Autodesk Inventor part; units mm, degrees
ref_plane "YZ Plane" through (0, 0, 0) normal (1, 0, 0) x (0, 1, 0)
ref_plane "XZ Plane" through (0, 0, 0) normal (0, 1, 0) x (-1, 0, 0)
ref_plane "XY Plane" through (0, 0, 0) normal (0, 0, 1) x (1, 0, 0)
sketch "スケッチ1" plane through (0, 0, 0) normal (0, 1, 0) x (-1, 0, 0)
  line L0 (7.5, -7.5) -> (-7.5, -7.5)
  line L1 (-7.5, -7.5) -> (-7.5, 7.5)
  line L2 (-7.5, 7.5) -> (7.5, 7.5)
  line L3 (7.5, 7.5) -> (7.5, -7.5)
  line L4 (7.5, -7.5) -> (-7.5, 7.5) construction
  line L5 (-7.5, -7.5) -> (7.5, 7.5) construction
  point P0 (0, 0)
  dimension "d0" = 15
  dimension "d1" = 15
extrude "押し出し1" add sketch "スケッチ1" along normal blind 140
shell "シェル1" thickness 1 removed faces 2 at (-2.5, 0, -2.5) at (-2.5, 140, -2.5)
sketch "スケッチ2" plane through (-7.5, 0, 7.5) normal (0, 0, 1) x (1, 0, 0)
  line L0 (15, 0) -> (0, 0)
  line L1 (0, 140) -> (15, 140)
  point P0 (7.5, 0)
  point P1 (7.5, 8)
  point P2 (7.5, 23)
  point P3 (7.5, 0)
  point P4 (7.5, 132)
  point P5 (7.5, 112)
  point P6 (7.5, 140)
  dimension "d5" = 8
  dimension "d6" = 15
  dimension "d14" = 8
  dimension "d15" = 20
hole "穴1" at (0, 8, 7.5) at (0, 23, 7.5) at (0, 132, 7.5) at (0, 112, 7.5) direction (0, 0, -1) diameter 3.2 end through all
sketch "スケッチ3" plane through (-7.5, 0, -7.5) normal (-1, 0, 0) x (0, 0, 1)
  line L0 (15, 0) -> (0, 0)
  point P0 (7.5, 0)
  point P1 (7.5, 37.5)
  point P2 (7.5, 102.5)
  point P3 (7.5, 0)
  point P4 (7.5, 0)
  dimension "d16" = 37.5
  dimension "d17" = 65
hole "穴2" at (-7.5, 37.5, 0) at (-7.5, 102.5, 0) direction (1, 0, 0) diameter 3.2 end through all
sketch "スケッチ4" plane through (-7.5, 0, 7.5) normal (0, 0, 1) x (1, 0, 0)
  circle A0 centre (94.8138, 137.4022) radius 1.6
  circle A1 centre (-2.6682, 183.8917) radius 1.6
  circle A2 centre (99.3065, 100.3608) radius 1.6
  circle A3 centre (1.8246, 146.8503) radius 1.6
  circle A4 centre (7.5, 112) radius 1.2295
  circle A5 centre (7.5, 132) radius 1.2295
  line L0 (112.2687, 136.8332) -> (109.5609, 138.1246)
  arc A6 (110.4218, 139.9298) -> (109.5609, 138.1246) centre (109.9914, 139.0272) ccw
  line L1 (110.4218, 139.9298) -> (112.1436, 143.5402)
  arc A7 (113.8704, 143.6762) -> (112.1436, 143.5402) centre (113.0463, 143.1098) ccw
  arc A8 (114.8515, 142.2489) -> (113.8704, 143.6762) centre (113.9489, 142.6793) ccw
  line L2 (114.8515, 142.2489) -> (113.1296, 138.6384)
  arc A9 (112.2687, 136.8332) -> (113.1296, 138.6384) centre (112.6992, 137.7358) ccw
  line L3 (120.017, 153.0802) -> (118.2951, 149.4697)
  arc A10 (116.5684, 149.3337) -> (118.2951, 149.4697) centre (117.3925, 149.9002) ccw
  arc A11 (115.5873, 150.7611) -> (116.5684, 149.3337) centre (116.4899, 150.3307) ccw
  line L4 (115.5873, 150.7611) -> (117.3091, 154.3716)
  arc A12 (118.1701, 156.1768) -> (117.3091, 154.3716) centre (117.7396, 155.2742) ccw
  line L5 (118.1701, 156.1768) -> (120.8779, 154.8854)
  arc A13 (120.017, 153.0802) -> (120.8779, 154.8854) centre (120.4474, 153.9828) ccw
  line L6 (106.2423, 124.1966) -> (103.5345, 125.488)
  arc A14 (104.3954, 127.2932) -> (103.5345, 125.488) centre (103.9649, 126.3906) ccw
  line L7 (104.3954, 127.2932) -> (106.1172, 130.9037)
  arc A15 (107.8439, 131.0397) -> (106.1172, 130.9037) centre (107.0198, 130.4732) ccw
  arc A16 (108.8251, 129.6123) -> (107.8439, 131.0397) centre (107.9225, 130.0428) ccw
  line L8 (108.8251, 129.6123) -> (107.1032, 126.0019)
  arc A17 (106.2423, 124.1966) -> (107.1032, 126.0019) centre (106.6728, 125.0992) ccw
  circle A18 centre (51.5477, 186.0658) radius 1.6
  circle A19 centre (60.463, 120.5473) radius 1.5
  circle A20 centre (40.987, 157.5329) radius 1.5
  circle A21 centre (30.2256, 134.9676) radius 1.5
  circle A22 centre (71.2245, 143.1126) radius 1.5
  circle A23 centre (72.3508, 176.2555) radius 1.25
  circle A24 centre (94.0134, 165.9245) radius 1.25
  arc A25 (80.796, 100.4622) -> (79.0196, 101.3811) centre (79.9078, 100.9217) ccw
  line L9 (80.796, 100.4622) -> (75.2827, 89.8038)
  arc A26 (73.5063, 90.7226) -> (75.2827, 89.8038) centre (74.3945, 90.2632) ccw
  line L10 (73.5063, 90.7226) -> (64.6242, 95.3171)
  arc A27 (62.8478, 96.2359) -> (64.6242, 95.3171) centre (63.736, 95.7765) ccw
  line L11 (62.8478, 96.2359) -> (68.3611, 106.8944)
  arc A28 (70.1375, 105.9755) -> (68.3611, 106.8944) centre (69.2493, 106.435) ccw
  line L12 (70.1375, 105.9755) -> (79.0196, 101.3811)
  circle A29 centre (28.7854, 103.2592) radius 1.5
  circle A30 centre (67.6869, 90.3552) radius 1.5
  circle A31 centre (75.9568, 106.343) radius 1.5
  circle A32 centre (31.7101, 121.02) radius 1.5
  line L13 (38.1296, 116.9224) -> (36.1798, 105.0819)
  arc A33 (34.2064, 105.4069) -> (36.1798, 105.0819) centre (35.1931, 105.2444) ccw
  line L14 (34.2064, 105.4069) -> (24.3393, 107.0317)
  arc A34 (22.3659, 107.3567) -> (24.3393, 107.0317) centre (23.3526, 107.1942) ccw
  line L15 (22.3659, 107.3567) -> (24.3157, 119.1972)
  arc A35 (26.2891, 118.8723) -> (24.3157, 119.1972) centre (25.3024, 119.0347) ccw
  line L16 (26.2891, 118.8723) -> (36.1562, 117.2474)
  arc A36 (38.1296, 116.9224) -> (36.1562, 117.2474) centre (37.1429, 117.0849) ccw
  circle A37 centre (-0.9114, 173.6368) radius 1.6
  circle A38 centre (91.1549, 129.73) radius 1.6
  arc A39 (89.211, 114.0386) -> (91.0163, 113.1777) centre (90.1137, 113.6081) ccw
  line L17 (89.211, 114.0386) -> (80.1849, 118.3432)
  arc A40 (78.3797, 119.2041) -> (80.1849, 118.3432) centre (79.2823, 118.7736) ccw
  line L18 (78.3797, 119.2041) -> (83.5452, 130.0354)
  arc A41 (85.3504, 129.1745) -> (83.5452, 130.0354) centre (84.4478, 129.605) ccw
  line L19 (85.3504, 129.1745) -> (94.3765, 124.8699)
  arc A42 (96.1818, 124.009) -> (94.3765, 124.8699) centre (95.2792, 124.4395) ccw
  line L20 (96.1818, 124.009) -> (91.0163, 113.1777)
  arc A43 (-6.7159, 173.0812) -> (-8.5211, 173.9421) centre (-7.6185, 173.5117) ccw
  line L21 (-6.7159, 173.0812) -> (2.3103, 168.7766)
  arc A44 (4.1155, 167.9157) -> (2.3103, 168.7766) centre (3.2129, 168.3462) ccw
  line L22 (4.1155, 167.9157) -> (-1.05, 157.0844)
  arc A45 (-2.8552, 157.9453) -> (-1.05, 157.0844) centre (-1.9526, 157.5148) ccw
  line L23 (-2.8552, 157.9453) -> (-11.8813, 162.2499)
  arc A46 (-13.6866, 163.1108) -> (-11.8813, 162.2499) centre (-12.784, 162.6803) ccw
  line L24 (-13.6866, 163.1108) -> (-8.5211, 173.9421)
  circle A47 centre (83.4066, 113.4831) radius 1.6
  circle A48 centre (-8.6597, 157.3898) radius 1.6
  circle A49 centre (9.0871, 193.022) radius 1.25
  circle A50 centre (11.8045, 158.4877) radius 1.25
  circle A51 centre (40.3533, 178.1082) radius 1.25
  circle A52 centre (60.4103, 159.3488) radius 1.2295
  circle A53 centre (78.2541, 161.9181) radius 1.2295
  circle A54 centre (51.1757, 174.8318) radius 1.2295
  arc A55 (-2.9, 96) -> (-6, 96) centre (-4.45, 96) ccw
  line L25 (-2.9, 96) -> (-2.9, 90)
  arc A56 (-6, 90) -> (-2.9, 90) centre (-4.45, 90) ccw
  line L26 (-6, 90) -> (-6, 96)
  circle A57 centre (49.5584, 72.8565) radius 1.6
  circle A58 centre (7.5, 59) radius 1.25
  circle A59 centre (7.5, 93) radius 1.25
  arc A60 (-2.9, 62) -> (-6, 62) centre (-4.45, 62) ccw
  line L27 (-2.9, 62) -> (-2.9, 56)
  arc A61 (-6, 56) -> (-2.9, 56) centre (-4.45, 56) ccw
  line L28 (-6, 56) -> (-6, 62)
  arc A62 (0, 103) -> (0, 106) centre (0, 104.5) ccw
  line L29 (-9, 103) -> (0, 103)
  line L30 (-9, 83) -> (-9, 103)
  line L31 (0, 83) -> (-9, 83)
  arc A63 (0, 80) -> (0, 83) centre (0, 81.5) ccw
  line L32 (0, 80) -> (0, 72)
  arc A64 (0, 69) -> (0, 72) centre (0, 70.5) ccw
  line L33 (-9, 69) -> (0, 69)
  line L34 (-9, 49) -> (-9, 69)
  line L35 (0, 49) -> (-9, 49)
  arc A65 (0, 46) -> (0, 49) centre (0, 47.5) ccw
  line L36 (0, 46) -> (0, 42)
  arc A66 (0, 42) -> (1.4237, 42.3594) centre (0, 45) ccw
  line L37 (1.4237, 42.3594) -> (101.4896, 96.3119)
  arc A67 (101.4896, 96.3119) -> (103.6033, 98.7183) centre (99.3065, 100.3608) ccw
  line L38 (124.1837, 152.5545) -> (103.6033, 98.7183)
  arc A68 (124.1837, 152.5545) -> (122.1359, 157.6089) centre (120.4474, 153.9828) ccw
  line L39 (53.2362, 189.6919) -> (122.1359, 157.6089)
  arc A69 (53.2362, 189.6919) -> (48.9495, 189.107) centre (51.5477, 186.0658) ccw
  line L40 (38.5483, 180.221) -> (48.9495, 189.107)
  arc A70 (38.5483, 180.221) -> (37.5746, 178.1426) centre (40.3533, 178.1082) ccw
  arc A71 (35.9884, 171.3281) -> (37.5746, 178.1426) centre (21.2759, 178.3445) ccw
  line L41 (35.9884, 171.3281) -> (35.1275, 169.5229)
  arc A72 (5.7024, 183.5558) -> (35.1275, 169.5229) centre (20.415, 176.5393) ccw
  line L42 (5.7024, 183.5558) -> (6.5633, 185.361)
  arc A73 (10.8623, 190.8844) -> (6.5633, 185.361) centre (21.2759, 178.3445) ccw
  arc A74 (10.8623, 190.8844) -> (7.898, 195.5334) centre (9.0871, 193.022) ccw
  line L43 (-5.2359, 189.3145) -> (7.898, 195.5334)
  arc A75 (-5.2359, 189.3145) -> (-8.284, 186.0042) centre (-2.6682, 183.8917) ccw
  line L44 (-16.5278, 164.0887) -> (-8.284, 186.0042)
  arc A76 (-16.5278, 164.0887) -> (-16.5876, 161.4424) centre (-12.784, 162.6803) ccw
  line L45 (-16.5876, 161.4424) -> (-0.1473, 110.9284)
  arc A77 (0, 110) -> (-0.1473, 110.9284) centre (-3, 110) ccw
  line L46 (0, 110) -> (0, 106)
  point P0 (7.5, 0)
hole "穴3" at (0, 59, 7.5) at (0, 93, 7.5) direction (0, 0, -1) diameter 3.2 end through all
properties part number "PitchSquarePipe2" material "アルミニウム 5005-H12"
Verification items for the finished model (mm, model axes). A direction names the side the tool comes from. Coordinates: 2 decimals unless noted, no trailing zeros. Write each loop counter-clockwise with the first axis right and the second up, starting at its lowest first coordinate (ties: lowest second). Pieces come first, ordered by that corner, then holes. Notation, with made-up numbers: M -10,28.25 L 15,28.25 A20 cw 15,61.25 Z; hole C 81,66.5 d8. An arc over 180 degrees is marked long. Use CSV: the item, a comma, the result in double quotes.
Q1. Section check C-C, the plane x = 4.75. Enter the section's corners in (y, z), and give its area (3 significant figures).
Computed values:
outline,"M 0,-7.5 L 140,-7.5 L 140,-6.5 L 0,-6.5 Z; M 0,6.5 L 140,6.5 L 140,7.5 L 0,7.5 Z"
area,"280 mm²"
Q2. Section check B-B, the plane z = 0. Enter the section's corners in (x, y), and give its area (3 significant figures).
Computed values:
outline,"M -7.5,0 L -6.5,0 L -6.5,35.9 L -7.5,35.9 Z; M -7.5,39.1 L -6.5,39.1 L -6.5,100.9 L -7.5,100.9 Z; M -7.5,104.1 L -6.5,104.1 L -6.5,140 L -7.5,140 Z; M 6.5,0 L 7.5,0 L 7.5,35.9 L 6.5,35.9 Z; M 6.5,39.1 L 7.5,39.1 L 7.5,100.9 L 6.5,100.9 Z; M 6.5,104.1 L 7.5,104.1 L 7.5,140 L 6.5,140 Z"
area,"267 mm²"
Q3. Go/stop test with a flat-tipped pin: P1, Ø1.9, axis at x = 0, y = 23, coming from the -Z side. Record where the tip stops, or that it passes through.
Computed values:
P1,"through"
Q4. Mould release check, pull along X, two halves, no side actions. Record for faces 3 (the flat face through (-7.5, 69, 0)), 4 (the cylindrical face through (0.61, 130.52, 6.99)), 5 (the flat face through (0, 69, 7.5)): pulls with the +X half, pulls with the -X half, needs draft (parallel to the pull), parting line crosses it, or undercut.
Computed values:
face 3,"pulls with the -X half"
face 4,"undercut"
face 5,"needs draft"
Q5. Thickness scan on line 1 along Z through (x, y) = (5.25, 109); line 2 along Z through (x, y) = (-7.1, 37.5). Record the ranges inside material, lowest first. Write a range as [from, to].
Computed values:
line 1,"[-7.5, -6.5], [6.5, 7.5]"
line 2,"[-7.5, -1.6], [1.6, 7.5]"
Q6. Set-up check for faces 1 (the flat face through (0, 69, -6.5)), 2 (the cylindrical face through (-0.07, 94.6, -7.01)): record each of +Z, -Z, +X, -X, +Y, -Y from which the full face is reachable in a straight line by a thin tool's end or side.
Computed values:
face 1,"+Y, -Y"
face 2,"+Z, -Z"
Q7. Section check A-A, the plane y = 23. Enter the section's corners in (x, z).
Computed values:
outline,"M -7.5,-7.5 L -1.6,-7.5 L -1.6,-6.5 L -6.5,-6.5 L -6.5,6.5 L -1.6,6.5 L -1.6,7.5 L -7.5,7.5 Z; M 1.6,-7.5 L 7.5,-7.5 L 7.5,7.5 L 1.6,7.5 L 1.6,6.5 L 6.5,6.5 L 6.5,-6.5 L 1.6,-6.5 Z"
